Could you check a few things on this model? Use its own coordinates, in mm. Coordinates: 2 decimals unless noted, no trailing zeros. Loops run counter-clockwise (first coordinate to the right, second up) from the corner with the lowest first, then second, coordinate; pieces in that order, holes last.
1) Will this pin go through, and if not, where does the flat tip stop? P1, Ø5, axis at y = 10, z = 130, coming from the -X side.
2) Imagine slicing it at C-C on y = 1.75. Please give me the cut outline in (x, z).
3) If I drill on line 1 along Z through (x, y) = (1.3, 10); line 2 along Y through (x, z) = (1.8, 130); line 3 along Z through (x, y) = (2.45, 14), over which ranges is the centre line in solid material (lowest first)?
4) Imagine slicing it at B-B on x = 1.15. Please give me the cut outline in (y, z), plus the area to 3 significant figures.
5) Imagine slicing it at A-A on y = 10. Please give me the cut outline in (x, z), plus the area to 3 significant figures.
Autodesk Inventor part; units mm, degrees
ref_plane "YZ Plane" through (0, 0, 0) normal (1, 0, 0) x (0, 1, 0)
ref_plane "XZ Plane" through (0, 0, 0) normal (0, 1, 0) x (-1, 0, 0)
ref_plane "XY Plane" through (0, 0, 0) normal (0, 0, 1) x (1, 0, 0)
sketch "Szkic1" plane through (0, 0, 0) normal (1, 0, 0) x (0, 1, 0)
  line L0 (10, 0) -> (10, 0)
  line L1 (20, 10) -> (20, 130)
  line L2 (10, 140) -> (10, 140)
  line L3 (0, 130) -> (0, 10)
  arc A0 (20, 130) -> (10, 140) centre (10, 130) ccw
  arc A1 (10, 140) -> (0, 130) centre (10, 130) ccw
  arc A2 (10, 0) -> (20, 10) centre (10, 10) ccw
  arc A3 (0, 10) -> (10, 0) centre (10, 10) ccw
  circle A4 centre (10, 130) radius 1.6
  circle A5 centre (10, 10) radius 1.6
  point P0 (0, 0)
  point P1 (20, 140)
  point P2 (0, 140)
  dimension "d0" = 20
  dimension "d1" = 10
  dimension "d2" = 10
  dimension "d3" = 10
  dimension "d4" = 10
  dimension "d5" = 3.2
  dimension "d6" = 3.2
  dimension "d7" = 120
extrude "Wyciągnięcie proste1" add sketch "Szkic1" along normal blind 3
properties part number "segment1"
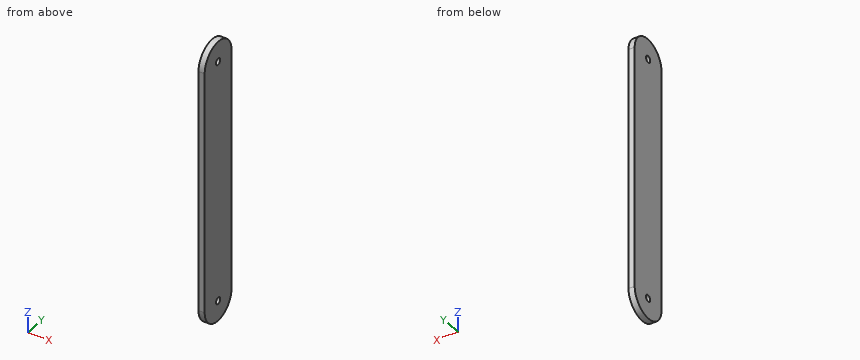
Filled in:
1. P1: stops at x = 0
2. outline: (0, 4.35) - (3, 4.35) - (3, 135.65) - (0, 135.65) - close
3. line 1: z = 0 to 8.4, 11.6 to 128.4, 131.6 to 140
3. line 2: y = 0 to 8.4, 11.6 to 20
3. line 3: z = 0.83 to 139.17
4. outline: (0, 10) arc R10 ccw to (20, 10) - (20, 130) arc R10 ccw to (0, 130) - close; hole circle Ø3.2 at (10, 10); hole circle Ø3.2 at (10, 130)
4. area: 2,700 mm2
5. outline: (0, 0) - (3, 0) - (3, 8.4) - (0, 8.4) - close; (0, 11.6) - (3, 11.6) - (3, 128.4) - (0, 128.4) - close; (0, 131.6) - (3, 131.6) - (3, 140) - (0, 140) - close
5. area: 401 mm2
